Read the model definition and answer for the solid it produces. Units are mm, in the model's axes. A direction names the side the tool comes from. Coordinates: 2 decimals unless noted, no trailing zeros. Order: outer loops, then holes, each group sorted by start corner. A loop starts at its lowest first (then second) coordinate and runs counter-clockwise, first axis right, second up. Notation, with made-up numbers: (73.25, 53.5) -> (122.25, 53.5) arc R22 cw to (122.25, 73.5) -> close; hole circle Ø6 at (58, -30.5). An arc over 180 degrees is marked (long way). Answer in a Markdown table with one row per item.
from build123d import *

# Parameters (mm, degrees)
CROQUIS1_R              = 11
CROQUIS1_R_2            = 1.55
SALIENTE_EXTRUIR1_DEPTH = 5.5
CROQUIS3_W              = 5.5
CROQUIS3_H              = 5
SALIENTE_EXTRUIR3_DEPTH = 3
CROQUIS6_W              = 3
CROQUIS6_H              = 3
CORTAR_EXTRUIR2_DEPTH   = 8
CROQUIS7_W              = 2.5
CROQUIS7_H              = 6
CORTAR_EXTRUIR3_DEPTH   = 6.5


with BuildPart() as part:
    # Croquis1 → Saliente-Extruir1 (new body)
    with BuildSketch(Plane.XY):
        Polygon((4, 0), (0, 4), (0, 38), (4, 42), (42, 42), (42, 0), align=None)
        with Locations((21, 21)):
            Circle(CROQUIS1_R, mode=Mode.SUBTRACT)
        with Locations((36.5, 36.5)):
            Circle(CROQUIS1_R_2, mode=Mode.SUBTRACT)
        with Locations((36.5, 5.5)):
            Circle(CROQUIS1_R_2, mode=Mode.SUBTRACT)
        with Locations((5.5, 5.5)):
            Circle(CROQUIS1_R_2, mode=Mode.SUBTRACT)
        with Locations((5.5, 36.5)):
            Circle(CROQUIS1_R_2, mode=Mode.SUBTRACT)
    extrude(amount=SALIENTE_EXTRUIR1_DEPTH)

    # Croquis3 → Saliente-Extruir3 (add)
    with BuildSketch(Plane(origin=(42, 0, 0), x_dir=(0, 0, -1), z_dir=(1, 0, 0))):
        with Locations((-2.75, 26.5)):
            Rectangle(CROQUIS3_W, CROQUIS3_H)
        with Locations((-2.75, 11.5)):
            Rectangle(CROQUIS3_W, CROQUIS3_H)
    extrude(amount=SALIENTE_EXTRUIR3_DEPTH)

    # Croquis6 → Cortar-Extruir2 (cut)
    with BuildSketch(Plane(origin=(42, 0, 0), x_dir=(0, 0, -1), z_dir=(1, 0, 0))):
        with Locations((-2.75, 19)):
            Rectangle(CROQUIS6_W, CROQUIS6_H)
    extrude(amount=-CORTAR_EXTRUIR2_DEPTH, mode=Mode.SUBTRACT)

    # Croquis7 → Cortar-Extruir3 (cut, through all)
    with BuildSketch(Plane.XY.offset(5.5)):
        with Locations((38.75, 19)):
            Rectangle(CROQUIS7_W, CROQUIS7_H)
    extrude(amount=-CORTAR_EXTRUIR3_DEPTH, mode=Mode.SUBTRACT)


solid = part.part
Q1. The part is cut by section A-A (x = 36.5). Write down the section's boundary in (y, z), then the cut area to 3 significant figures.
Outcome:
| item | result |
|---|---|
| outline | (0, 0) -> (3.95, 0) -> (3.95, 5.5) -> (0, 5.5) -> close; (7.05, 0) -> (34.95, 0) -> (34.95, 5.5) -> (7.05, 5.5) -> close; (38.05, 0) -> (42, 0) -> (42, 5.5) -> (38.05, 5.5) -> close; hole (17.5, 1.25) -> (20.5, 1.25) -> (20.5, 4.25) -> (17.5, 4.25) -> close |
| area | 188 mm² |
Q2. For faces 1 (the face through (41, 20.5, 3)), 2 (the face through (37.5, 19, 1)), 3 (the face through (43, 29, 3)), determine the directions among +Z, -Z, +X, -X, +Y, -Y from which every point of the face is accessible in a straight line to the end or side of a thin tool.
Outcome:
| item | result |
|---|---|
| face 1 | +X |
| face 2 | +Z, -Z |
| face 3 | +Z, -Z, +X, +Y |
Q3. For a pull along X with two mould halves and no side action, classify faces 4 (the face through (31.161, 16.787, 2.712)), 5 (the face through (2, 2, 3)), 6 (the face through (39, 16, 3)), 7 (the face through (43, 24, 3)) as pulls with the +X half, pulls with the -X half, needs draft (parallel to the pull), parting line crosses it, or undercut.
Outcome:
| item | result |
|---|---|
| face 4 | undercut |
| face 5 | pulls with the -X half |
| face 6 | undercut |
| face 7 | needs draft |
Q4. Given pin 1 (1.6 mm diameter, centred on y = 19, z = 3, fed in from +X); pin 2 (8 mm diameter, centred on x = 20, y = 17, fed in from +Z); pin 3 (0.9 mm diameter, centred on x = 43, z = 4, fed in from +Y); pin 4 (2.5 mm diameter, centred on y = 18.5, z = 2.5, fed in from +X), each flat-ended and moving along its own axis, determine where each tip first touches the part or whether it passes through.
Outcome:
| item | result |
|---|---|
| pin 1 | x = 34 |
| pin 2 | through |
| pin 3 | y = 29 |
| pin 4 | x = 42 |
Q5. The part is cut by section B-B (z = 3.15). Give the number of separate pieces and of enclosed holes in the cut face, then the cut area to 3 significant figures.
Outcome:
| item | result |
|---|---|
| separate pieces | 1 |
| enclosed holes | 5 |
| area | 1,340 mm² |
Q6. The part is cut by section C-C (x = 5.5). Write down the section's boundary in (y, z), then the cut area to 3 significant figures.
Outcome:
| item | result |
|---|---|
| outline | (0, 0) -> (3.95, 0) -> (3.95, 5.5) -> (0, 5.5) -> close; (7.05, 0) -> (34.95, 0) -> (34.95, 5.5) -> (7.05, 5.5) -> close; (38.05, 0) -> (42, 0) -> (42, 5.5) -> (38.05, 5.5) -> close |
| area | 197 mm² |
Q7. Consider line 1 (Y direction, x = 5.5, z = 1.8); line 2 (Y direction, x = 41.5, z = 1.95); line 3 (Y direction, x = 21.5, z = 0.6). Determine where each line is inside the solid, lowest interval first.
Outcome:
| item | result |
|---|---|
| line 1 | 0 to 3.95, 7.05 to 34.95, 38.05 to 42 |
| line 2 | 0 to 17.5, 20.5 to 42 |
| line 3 | 0 to 10.01, 31.99 to 42 |
